from build123d import *

# Parameters (mm, degrees)
F0_W          = 51.5
F0_H          = 51.5
F1_DEPTH      = 40
F2_DEPTH      = 35
F0_R          = 6
F3_DEPTH      = 2
F4_T4_DEPTH   = 7.1433659759
F4_T10_DEPTH  = 7.1433659759
F4_T16_DEPTH  = 7.1433659759
F4_T22_DEPTH  = 7.1433659759
F4_T28_DEPTH  = 7.1433659759
F4_T34_DEPTH  = 7.1433659759
F4_T40_DEPTH  = 7.1433659759
F4_T46_DEPTH  = 7.1433659759
F4_T49_DEPTH  = 46.5
F4_T51_DEPTH  = 46.5
F4_T53_DEPTH  = 56.6433659759
F4_T55_DEPTH  = 56.6433659759
F4_T63_DEPTH  = 49.071682988
F4_T67_DEPTH  = 49.071682988
F4_T74_DEPTH  = 49.071682988
F4_T78_DEPTH  = 49.071682988
F4_T85_DEPTH  = 49.071682988
F4_T89_DEPTH  = 49.071682988
F4_T96_DEPTH  = 49.071682988
F4_T100_DEPTH = 49.071682988


# Not quite as in the source:
# - a fillet or chamfer that OpenCascade refuses, or shapes differently, is made with other operations: its cross-section is extruded or revolved along the edge and cut away or added


with BuildPart() as f1:
    # F0 (on Top) → F1 (new body)
    with BuildSketch(Plane.XY):
        Rectangle(F0_W, F0_H)
        Polygon((-23.25, 17.25), (-23.25, 23.25), (-17.25, 23.25), (-15.25, 23.25), (15.25, 23.25), (17.25, 23.25), (23.25, 23.25), (23.25, 17.25), (23.25, 15.25), (23.25, -15.25), (23.25, -17.25), (23.25, -23.25), (17.25, -23.25), (15.25, -23.25), (-15.25, -23.25), (-17.25, -23.25), (-23.25, -23.25), (-23.25, -17.25), (-23.25, -15.25), (-23.25, 15.25), align=None, mode=Mode.SUBTRACT)
    extrude(amount=F1_DEPTH)

    # F0 (on Top) → F2 (join)
    with BuildSketch(Plane.XY):
        Rectangle(F0_W, F0_H)
        Polygon((-23.25, 17.25), (-23.25, 23.25), (-17.25, 23.25), (-15.25, 23.25), (15.25, 23.25), (17.25, 23.25), (23.25, 23.25), (23.25, 17.25), (23.25, 15.25), (23.25, -15.25), (23.25, -17.25), (23.25, -23.25), (17.25, -23.25), (15.25, -23.25), (-15.25, -23.25), (-17.25, -23.25), (-23.25, -23.25), (-23.25, -17.25), (-23.25, -15.25), (-23.25, 15.25), align=None, mode=Mode.SUBTRACT)
        Polygon((-22.45, 16.25), (-23.25, 17.25), (-23.25, 15.25), align=None)
        Polygon((-15.25, 23.25), (-17.25, 23.25), (-16.25, 22.45), align=None)
        Polygon((17.25, 23.25), (15.25, 23.25), (16.25, 22.45), align=None)
        Polygon((23.25, 15.25), (23.25, 17.25), (22.45, 16.25), align=None)
        Polygon((23.25, -17.25), (23.25, -15.25), (22.45, -16.25), align=None)
        Polygon((16.25, -22.45), (15.25, -23.25), (17.25, -23.25), align=None)
        Polygon((-16.25, -22.45), (-17.25, -23.25), (-15.25, -23.25), align=None)
        Polygon((-22.45, -16.25), (-23.25, -15.25), (-23.25, -17.25), align=None)
    extrude(amount=F2_DEPTH)

    # F0 (on Top) → F3 (join)
    with BuildSketch(Plane.XY):
        Polygon((-17.25, 23.25), (-23.25, 23.25), (-23.25, 17.25), (-22.45, 16.25), (-23.25, 15.25), (-23.25, -15.25), (-22.45, -16.25), (-23.25, -17.25), (-23.25, -23.25), (-17.25, -23.25), (-16.25, -22.45), (-15.25, -23.25), (15.25, -23.25), (16.25, -22.45), (17.25, -23.25), (23.25, -23.25), (23.25, -17.25), (22.45, -16.25), (23.25, -15.25), (23.25, 15.25), (22.45, 16.25), (23.25, 17.25), (23.25, 23.25), (17.25, 23.25), (16.25, 22.45), (15.25, 23.25), (-15.25, 23.25), (-16.25, 22.45), align=None)
        Circle(F0_R, mode=Mode.SUBTRACT)
    extrude(amount=F3_DEPTH)

    # F4: chamfer of 1 on 17 edges, made by hand


with BuildPart() as f4_tool2:
    # F4_s3 → F4_t4 (new body)
    with BuildSketch(Plane.YZ.offset(12.678317012)):
        Polygon((23.25, 36), (22.25, 35), (23.25, 35), align=None)
    extrude(amount=F4_T4_DEPTH)

    split(bisect_by=Plane(origin=(17.2926829268, 21.6158536585, 0), x_dir=(0, 0, 1), z_dir=(0.6246950476, 0.7808688094, 0)), keep=Keep.TOP)

    split(bisect_by=Plane(origin=(-4.6097560976, 5.762195122, 0), x_dir=(0, 0, 1), z_dir=(-0.6246950476, 0.7808688094, 0)), keep=Keep.TOP)


with BuildPart() as f1_1:
    add(f1.part)

    # F4_t1: union F4_tool2
    add(f4_tool2.part)


with BuildPart() as f4_tool8:
    # F4_s9 → F4_t10 (new body)
    with BuildSketch(Plane.YZ.offset(-19.821682988)):
        Polygon((23.25, 36), (22.25, 35), (23.25, 35), align=None)
    extrude(amount=F4_T10_DEPTH)

    split(bisect_by=Plane(origin=(4.6097560976, 5.762195122, 0), x_dir=(0, 0, 1), z_dir=(0.6246950476, 0.7808688094, 0)), keep=Keep.TOP)

    split(bisect_by=Plane(origin=(-17.2926829268, 21.6158536585, 0), x_dir=(0, 0, 1), z_dir=(-0.6246950476, 0.7808688094, 0)), keep=Keep.TOP)


with BuildPart() as f1_2:
    add(f1_1.part)

    # F4_t7: union F4_tool8
    add(f4_tool8.part)


with BuildPart() as f4_tool14:
    # F4_s15 → F4_t16 (new body)
    with BuildSketch(Plane.XZ.offset(12.678317012)):
        Polygon((23.25, 36), (22.25, 35), (23.25, 35), align=None)
    extrude(amount=F4_T16_DEPTH)

    split(bisect_by=Plane(origin=(21.6158536585, -17.2926829268, 0), x_dir=(0, 0, 1), z_dir=(0.7808688094, -0.6246950476, 0)), keep=Keep.TOP)

    split(bisect_by=Plane(origin=(5.762195122, 4.6097560976, 0), x_dir=(0, 0, 1), z_dir=(0.7808688094, 0.6246950476, 0)), keep=Keep.TOP)


with BuildPart() as f1_3:
    add(f1_2.part)

    # F4_t13: union F4_tool14
    add(f4_tool14.part)


with BuildPart() as f4_tool20:
    # F4_s21 → F4_t22 (new body)
    with BuildSketch(Plane.XZ.offset(-19.821682988)):
        Polygon((23.25, 36), (22.25, 35), (23.25, 35), align=None)
    extrude(amount=F4_T22_DEPTH)

    split(bisect_by=Plane(origin=(5.762195122, -4.6097560976, 0), x_dir=(0, 0, 1), z_dir=(0.7808688094, -0.6246950476, 0)), keep=Keep.TOP)

    split(bisect_by=Plane(origin=(21.6158536585, 17.2926829268, 0), x_dir=(0, 0, 1), z_dir=(0.7808688094, 0.6246950476, 0)), keep=Keep.TOP)


with BuildPart() as f1_4:
    add(f1_3.part)

    # F4_t19: union F4_tool20
    add(f4_tool20.part)


with BuildPart() as f4_tool26:
    # F4_s27 → F4_t28 (new body)
    with BuildSketch(Plane.XZ.offset(-12.678317012)):
        Polygon((-23.25, 36), (-22.25, 35), (-23.25, 35), align=None)
    extrude(amount=-F4_T28_DEPTH)

    split(bisect_by=Plane(origin=(-21.6158536585, 17.2926829268, 0), x_dir=(0, 0, 1), z_dir=(-0.7808688094, 0.6246950476, 0)), keep=Keep.TOP)

    split(bisect_by=Plane(origin=(-5.762195122, -4.6097560976, 0), x_dir=(0, 0, 1), z_dir=(-0.7808688094, -0.6246950476, 0)), keep=Keep.TOP)


with BuildPart() as f1_5:
    add(f1_4.part)

    # F4_t25: union F4_tool26
    add(f4_tool26.part)


with BuildPart() as f4_tool32:
    # F4_s33 → F4_t34 (new body)
    with BuildSketch(Plane.XZ.offset(19.821682988)):
        Polygon((-23.25, 36), (-22.25, 35), (-23.25, 35), align=None)
    extrude(amount=-F4_T34_DEPTH)

    split(bisect_by=Plane(origin=(-5.762195122, 4.6097560976, 0), x_dir=(0, 0, 1), z_dir=(-0.7808688094, 0.6246950476, 0)), keep=Keep.TOP)

    split(bisect_by=Plane(origin=(-21.6158536585, -17.2926829268, 0), x_dir=(0, 0, 1), z_dir=(-0.7808688094, -0.6246950476, 0)), keep=Keep.TOP)


with BuildPart() as f1_6:
    add(f1_5.part)

    # F4_t31: union F4_tool32
    add(f4_tool32.part)


with BuildPart() as f4_tool38:
    # F4_s39 → F4_t40 (new body)
    with BuildSketch(Plane.YZ.offset(-12.678317012)):
        Polygon((-23.25, 36), (-22.25, 35), (-23.25, 35), align=None)
    extrude(amount=-F4_T40_DEPTH)

    split(bisect_by=Plane(origin=(-17.2926829268, -21.6158536585, 0), x_dir=(0, 0, 1), z_dir=(-0.6246950476, -0.7808688094, 0)), keep=Keep.TOP)

    split(bisect_by=Plane(origin=(4.6097560976, -5.762195122, 0), x_dir=(0, 0, 1), z_dir=(0.6246950476, -0.7808688094, 0)), keep=Keep.TOP)


with BuildPart() as f1_7:
    add(f1_6.part)

    # F4_t37: union F4_tool38
    add(f4_tool38.part)


with BuildPart() as f4_tool44:
    # F4_s45 → F4_t46 (new body)
    with BuildSketch(Plane.YZ.offset(19.821682988)):
        Polygon((-23.25, 36), (-22.25, 35), (-23.25, 35), align=None)
    extrude(amount=-F4_T46_DEPTH)

    split(bisect_by=Plane(origin=(-4.6097560976, -5.762195122, 0), x_dir=(0, 0, 1), z_dir=(-0.6246950476, -0.7808688094, 0)), keep=Keep.TOP)

    split(bisect_by=Plane(origin=(17.2926829268, -21.6158536585, 0), x_dir=(0, 0, 1), z_dir=(0.6246950476, -0.7808688094, 0)), keep=Keep.TOP)


with BuildPart() as f1_8:
    add(f1_7.part)

    # F4_t43: union F4_tool44
    add(f4_tool44.part)

    # F4_s50 → F4_t49 (cut)
    with BuildSketch(Plane.YZ.offset(-23.25)):
        Polygon((24.25, 40), (23.25, 39), (23.25, 40), align=None)
        Polygon((-24.25, 40), (-23.25, 39), (-23.25, 40), align=None)
    extrude(amount=F4_T49_DEPTH, mode=Mode.SUBTRACT)

    # F4_s52 → F4_t51 (cut)
    with BuildSketch(Plane.XZ.offset(-23.25)):
        Polygon((-24.25, 40), (-23.25, 39), (-23.25, 40), align=None)
        Polygon((24.25, 40), (23.25, 39), (23.25, 40), align=None)
    extrude(amount=F4_T51_DEPTH, mode=Mode.SUBTRACT)

    # F4_s54 → F4_t53 (cut)
    with BuildSketch(Plane.YZ.offset(-28.321682988)):
        Polygon((25.75, 1), (24.75, 0), (25.75, 0), align=None)
        Polygon((-25.75, 1), (-24.75, 0), (-25.75, 0), align=None)
    extrude(amount=F4_T53_DEPTH, mode=Mode.SUBTRACT)

    # F4_s56 → F4_t55 (cut)
    with BuildSketch(Plane.XZ.offset(-28.321682988)):
        Polygon((-25.75, 1), (-24.75, 0), (-25.75, 0), align=None)
        Polygon((25.75, 1), (24.75, 0), (25.75, 0), align=None)
    extrude(amount=F4_T55_DEPTH, mode=Mode.SUBTRACT)

    # F4_s57 → F4_t58 (revolve, cut)
    with BuildSketch(Plane.XZ):
        Polygon((6, 1), (7, 0), (6, 0), align=None)
    revolve(axis=Axis((0, 0, 0), (0, 0, 1)), mode=Mode.SUBTRACT)


with BuildPart() as f4_tool61:
    # F4_s62 → F4_t63 (new body)
    with BuildSketch(Plane.YZ.offset(25.821682988)):
        Polygon((24.25, 40), (23.25, 39), (23.25, 40), align=None)
    extrude(amount=-F4_T63_DEPTH)

    split(bisect_by=Plane.YZ.offset(23.25), keep=Keep.TOP)


with BuildPart() as f4_tool65:
    # F4_s66 → F4_t67 (new body)
    with BuildSketch(Plane.XZ.offset(23.25)):
        Polygon((24.25, 40), (23.25, 39), (23.25, 40), align=None)
    extrude(amount=-F4_T67_DEPTH)

    split(bisect_by=Plane.XZ.offset(-23.25), keep=Keep.BOTTOM)


with BuildPart() as f4_tool61_1:
    add(f4_tool61.part)

    # F4_t69: intersect F4_tool65
    add(f4_tool65.part, mode=Mode.INTERSECT)


with BuildPart() as f1_9:
    add(f1_8.part)

    # F4_t59: cut F4_tool61
    add(f4_tool61_1.part, mode=Mode.SUBTRACT)


with BuildPart() as f4_tool72:
    # F4_s73 → F4_t74 (new body)
    with BuildSketch(Plane.XZ.offset(-25.821682988)):
        Polygon((-24.25, 40), (-23.25, 39), (-23.25, 40), align=None)
    extrude(amount=F4_T74_DEPTH)

    split(bisect_by=Plane.XZ.offset(-23.25), keep=Keep.BOTTOM)


with BuildPart() as f4_tool76:
    # F4_s77 → F4_t78 (new body)
    with BuildSketch(Plane.YZ.offset(23.25)):
        Polygon((24.25, 40), (23.25, 39), (23.25, 40), align=None)
    extrude(amount=-F4_T78_DEPTH)

    split(bisect_by=Plane.YZ.offset(-23.25), keep=Keep.BOTTOM)


with BuildPart() as f4_tool72_1:
    add(f4_tool72.part)

    # F4_t80: intersect F4_tool76
    add(f4_tool76.part, mode=Mode.INTERSECT)


with BuildPart() as f1_10:
    add(f1_9.part)

    # F4_t70: cut F4_tool72
    add(f4_tool72_1.part, mode=Mode.SUBTRACT)


with BuildPart() as f4_tool83:
    # F4_s84 → F4_t85 (new body)
    with BuildSketch(Plane.XZ.offset(-23.25)):
        Polygon((-24.25, 40), (-23.25, 39), (-23.25, 40), align=None)
    extrude(amount=F4_T85_DEPTH)

    split(bisect_by=Plane.XZ.offset(23.25), keep=Keep.TOP)


with BuildPart() as f4_tool87:
    # F4_s88 → F4_t89 (new body)
    with BuildSketch(Plane.YZ.offset(-25.821682988)):
        Polygon((-24.25, 40), (-23.25, 39), (-23.25, 40), align=None)
    extrude(amount=F4_T89_DEPTH)

    split(bisect_by=Plane.YZ.offset(-23.25), keep=Keep.BOTTOM)


with BuildPart() as f4_tool83_1:
    add(f4_tool83.part)

    # F4_t91: intersect F4_tool87
    add(f4_tool87.part, mode=Mode.INTERSECT)


with BuildPart() as f1_11:
    add(f1_10.part)

    # F4_t81: cut F4_tool83
    add(f4_tool83_1.part, mode=Mode.SUBTRACT)


with BuildPart() as f4_tool94:
    # F4_s95 → F4_t96 (new body)
    with BuildSketch(Plane.XZ.offset(25.821682988)):
        Polygon((24.25, 40), (23.25, 39), (23.25, 40), align=None)
    extrude(amount=-F4_T96_DEPTH)

    split(bisect_by=Plane.XZ.offset(23.25), keep=Keep.TOP)


with BuildPart() as f4_tool98:
    # F4_s99 → F4_t100 (new body)
    with BuildSketch(Plane.YZ.offset(-23.25)):
        Polygon((-24.25, 40), (-23.25, 39), (-23.25, 40), align=None)
    extrude(amount=F4_T100_DEPTH)

    split(bisect_by=Plane.YZ.offset(23.25), keep=Keep.TOP)


with BuildPart() as f4_tool94_1:
    add(f4_tool94.part)

    # F4_t102: intersect F4_tool98
    add(f4_tool98.part, mode=Mode.INTERSECT)


with BuildPart() as f1_12:
    add(f1_11.part)

    # F4_t92: cut F4_tool94
    add(f4_tool94_1.part, mode=Mode.SUBTRACT)


solid = f1_12.part
Geometry check sheet. Reference: the model listing, model coordinates, mm. A direction names the side the tool comes from. Give positions to 0.01 mm unless a question says otherwise; leave off trailing zeros. Loops run counter-clockwise (first coordinate to the right, second up) from the corner with the lowest first, then second, coordinate; pieces in that order, holes last. Notation, with made-up numbers: (3, 76.5) -> (13, 76.5) arc R12 ccw to (13, 89.5) -> close; hole circle Ø7 at (-24.5, -31). An arc over 180 degrees is marked (long way). Answer in a Markdown table with one row per item. Add a question column.
1) Draft check along Y on faces 1 (the face through (0, -25.75, 20)), 2 (the face through (0, -23.25, 20)), 3 (the face through (-25.75, 0, 20)). Enter one of: pulls with the +Y half, pulls with the -Y half, needs draft (parallel to the pull), parting line crosses it, or undercut.
2) Gauge pin test, flat ends, axial feed: P1, Ø8, axis at x = 11, y = -19.5, coming from the -Z side; P2, Ø1.5, axis at x = -15.5, y = -17.5, coming from the +Z side. Record the tip position at first contact, or that the pin passes through.
3) Material ranges on probe 1 along X at (y, z) = (-2.5, 6.5); probe 2 along Y at (x, z) = (0, 1), recorded low to high. Write a range as from..to.
4) Cross-section at A-A on y = 0. Record the boundary of the cut face in (x, z), and give its area (3 significant figures).
5) Cross-section at D-D on y = -19. Record the boundary of the cut face in (x, z).
6) Set-up check for faces 4 (the face through (-5, 5, 2)), 5 (the face through (25.75, 0, 20)): record each of +Z, -Z, +X, -X, +Y, -Y from which the full face is reachable in a straight line by a thin tool's end or side.
Outcome:
| question | item | result |
|---|---|---|
| 1 | face 1 | pulls with the -Y half |
| 1 | face 2 | undercut |
| 1 | face 3 | needs draft |
| 2 | P1 | stops at z = 0 |
| 2 | P2 | stops at z = 2 |
| 3 | probe 1 | x = -25.75..-23.25, 23.25..25.75 |
| 3 | probe 2 | y = -25.75..-6, 6..25.75 |
| 4 | outline | (-25.75, 1) -> (-24.75, 0) -> (-7, 0) -> (-6, 1) -> (-6, 2) -> (-23.25, 2) -> (-23.25, 39) -> (-24.25, 40) -> (-25.75, 40) -> close; (6, 1) -> (7, 0) -> (24.75, 0) -> (25.75, 1) -> (25.75, 40) -> (24.25, 40) -> (23.25, 39) -> (23.25, 2) -> (6, 2) -> close |
| 4 | area | 266 mm^2 |
| 5 | outline | (-25.75, 1) -> (-24.75, 0) -> (24.75, 0) -> (25.75, 1) -> (25.75, 40) -> (24.25, 40) -> (23.25, 39) -> (23.25, 2) -> (-23.25, 2) -> (-23.25, 39) -> (-24.25, 40) -> (-25.75, 40) -> close |
| 6 | face 4 | +Z |
| 6 | face 5 | +Z, -Z, +X, +Y, -Y |
